Here's how the part is built. I have some questions about the finished solid (model axes, mm). Face numbers are marked on the shaded views. A direction names the side the tool comes from. Coordinates: 2 decimals unless noted, no trailing zeros. Write each loop counter-clockwise with the first axis right and the second up, starting at its lowest first coordinate (ties: lowest second). Pieces come first, ordered by that corner, then holes.
(1) Thinking about a two-plate mould opening in Z: for the marked faces 1, 2 and 3, which applies, released by +Z, released by -Z, zero draft, split by the parting line, or undercut?
(2) Please list where these lines run through material, in increasing order: probe 1 along X at (y, z) = (25, 31.2); probe 2 along Z at (x, y) = (-1, 24); probe 3 along Z at (x, y) = (-24, 35).
(3) Which directions (+Z, -Z, +X, -X, +Y, -Y) give clear straight access to the entire face, cutting with the end or side of a thin tool? Please do the marked faces 4, 5, 6 and 7.
(4) Imagine slicing it at C-C, the plane x = 14. List the corners of the cut face in (y, z) for me.
(5) Imagine slicing it at A-A, the plane x = 22. List the corners of the cut face in (y, z) for me.
(6) For pin 1 Ø24 at (x, y) = (6.5, 24.5) entering from -Z; pin 2 Ø4 at (x, z) = (-10, -23) entering from +Y; pin 3 Ø3 at (x, y) = (17, 1.5) entering from -Z (3 decimals); pin 4 Ø25 at (y, z) = (39, -11.5) entering from +X, each with a flat end and sliding along its axis, tell me the tip position at first contact or that it passes through.
(7) Imagine slicing it at D-D, the plane y = 31. List the corners of the cut face in (x, z) for me.
(8) Imagine slicing it at B-B, the plane z = 5. List the corners of the cut face in (x, y) for me.
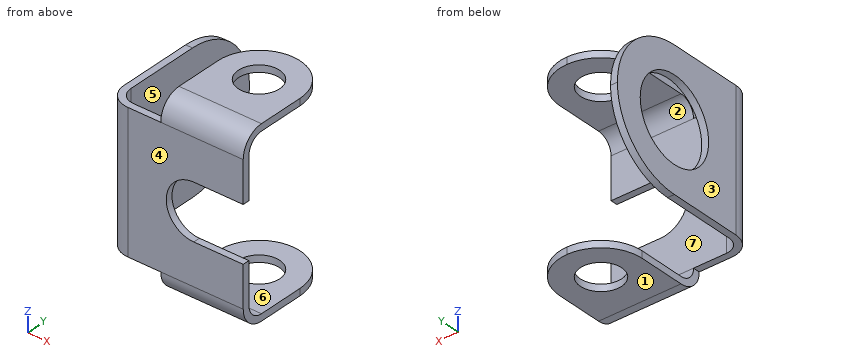
```python
from build123d import *

# Parameters (mm, degrees)
SKETCH1_W                    = 50
SKETCH1_H                    = 50
BASE_FLANGE1_DEPTH           = 2.5
EDGE_FLANGE1_STRIP_W         = 21
EDGE_FLANGE1_STRIP_H         = 2.5
EDGE_FLANGE1_STRIP_CUT_DEPTH = 50
EDGE_FLANGE1_DEPTH           = 50
BREAK_CORNER1_START          = -25
BREAK_CORNER1_DEPTH          = 2.5
SKETCH9_R                    = 15
CUT_EXTRUDE1_DEPTH           = 10
EDGE_FLANGE2_DEPTH           = 30
BREAK_CORNER2_START          = -33
BREAK_CORNER2_DEPTH          = 66
CUT_EXTRUDE2_DEPTH           = 93.633687177
CUT_EXTRUDE2_DEPTH_BACK      = 93.633687177
SKETCH13_R                   = 7.5
CUT_EXTRUDE3_DEPTH           = 71.853722556
CUT_EXTRUDE3_DEPTH_BACK      = 71.853722556


# Read off the part's stored shape, not the designer's step: Break-Corner1, Break-Corner2
# Sheet-metal steps are written as plain solids
with BuildPart() as part:
    # Sketch1 → Base-Flange1 (new body)
    with BuildSketch(Plane(origin=(0, 0, 0), x_dir=(1, 0, 0), z_dir=(0, 1, 0))):
        Rectangle(SKETCH1_W, SKETCH1_H)
    extrude(amount=BASE_FLANGE1_DEPTH)

    # Edge-Flange1 strip (across the edge) → Edge-Flange1 strip cut (cut)
    with BuildSketch(Plane(origin=(-25, 2.5, -25), x_dir=(1, 0, 0), z_dir=(0, 0, 1))):
        with Locations((-2.5, -1.25)):
            Rectangle(EDGE_FLANGE1_STRIP_W, EDGE_FLANGE1_STRIP_H)
    extrude(amount=EDGE_FLANGE1_STRIP_CUT_DEPTH, mode=Mode.SUBTRACT)

    # Edge-Flange1 section (across the edge) → Edge-Flange1 (add)
    with BuildSketch(Plane(origin=(-25, 2.5, -25), x_dir=(1, 0, 0), z_dir=(0, 0, 1))):
        with BuildLine():
            Line((0, 5.5), (0, 57.5))
            Line((0, 57.5), (2.5, 57.5))
            Line((2.5, 57.5), (2.5, 5.5))
            ThreePointArc((2.5, 5.5), (4.110912703, 1.610912703), (8, 0))
            Line((8, 0), (8, -2.5))
            ThreePointArc((8, -2.5), (2.343145751, -0.156854249), (0, 5.5))
        make_face()
    extrude(amount=EDGE_FLANGE1_DEPTH)

    # Break-Corner1 outline → Break-Corner1 (cut)
    with BuildSketch(Plane.YZ.offset(BREAK_CORNER1_START)):
        with BuildLine():
            Line((60, -25), (60, 0))
            ThreePointArc((60, 0), (52.67766953, -17.67766953), (35, -25))
            Line((35, -25), (60, -25))
        make_face()
        with BuildLine():
            ThreePointArc((35, 25), (52.67766953, 17.67766953), (60, 0))
            Line((60, 0), (60, 25))
            Line((60, 25), (35, 25))
        make_face()
    extrude(amount=BREAK_CORNER1_DEPTH, mode=Mode.SUBTRACT)

    # Sketch9 → Cut-Extrude1 (cut)
    with BuildSketch(Plane(origin=(-22.5, 0, 0), x_dir=(0, 0, -1), z_dir=(1, 0, 0))):
        with Locations(Location((0, 35, 0), (0, 0, 90))):
            Circle(SKETCH9_R)
    extrude(amount=-CUT_EXTRUDE1_DEPTH, mode=Mode.SUBTRACT)

    # Edge-Flange2 section (across the edge) → Edge-Flange2 (add)
    with BuildSketch(Plane(origin=(-5, 2.5, 30.5), x_dir=(0, 0, -1), z_dir=(1, 0, 0))):
        with BuildLine():
            Line((-2.5, 5.5), (-2.5, 37.5))
            Line((-2.5, 37.5), (0, 37.5))
            Line((0, 37.5), (0, 5.5))
            ThreePointArc((0, 5.5), (1.610912703, 1.610912703), (5.5, 0))
            Line((5.5, 0), (5.5, -2.5))
            ThreePointArc((5.5, -2.5), (-0.156854249, -0.156854249), (-2.5, 5.5))
        make_face()
    edge_flange2 = extrude(amount=EDGE_FLANGE2_DEPTH)

    # Mirror1: Edge-Flange2 across plane
    add(edge_flange2.mirror(Plane.XY))

    # Break-Corner2 outline → Break-Corner2 (cut)
    with BuildSketch(Plane.XY.offset(BREAK_CORNER2_START)):
        with BuildLine():
            ThreePointArc((-5, 25), (-0.606601718, 35.606601718), (10, 40))
            Line((10, 40), (-5, 40))
            Line((-5, 40), (-5, 25))
        make_face()
        with BuildLine():
            ThreePointArc((10, 40), (20.606601718, 35.606601718), (25, 25))
            Line((25, 25), (25, 40))
            Line((25, 40), (10, 40))
        make_face()
    extrude(amount=BREAK_CORNER2_DEPTH, mode=Mode.SUBTRACT)

    # Sketch13 → Cut-Extrude2 (cut, two sides: drawn at the far end of the back side and taken through both)
    with BuildSketch(Plane(origin=(0, 0, -33), x_dir=(-1, 0, 0), z_dir=(0, 0, -1)).offset(-CUT_EXTRUDE2_DEPTH_BACK)):
        with Locations(Location((-10, 25, 0), (0, 0, 90))):
            Circle(SKETCH13_R)
    extrude(amount=CUT_EXTRUDE2_DEPTH + CUT_EXTRUDE2_DEPTH_BACK, mode=Mode.SUBTRACT)

    # Sketch14 → Cut-Extrude3 (cut, two sides: drawn at the far end of the back side and taken through both)
    with BuildSketch(Plane(origin=(0, 2.5, 0), x_dir=(1, 0, 0), z_dir=(0, 1, 0)).offset(-CUT_EXTRUDE3_DEPTH_BACK)):
        with BuildLine():
            Line((7, 10), (37.302325581, 10))
            ThreePointArc((37.302325581, 10), (47.302325581, 0), (37.302325581, -10))
            Line((37.302325581, -10), (7, -10))
            ThreePointArc((7, -10), (-3, 0), (7, 10))
        make_face()
    extrude(amount=CUT_EXTRUDE3_DEPTH + CUT_EXTRUDE3_DEPTH_BACK, mode=Mode.SUBTRACT)


solid = part.part
```
Recorded:
1. face 1: released by -Z
1. face 2: undercut
1. face 3: zero draft
2. probe 1: x = -5 to 2.5, 17.5 to 25
2. probe 2: z = -33 to -30.5, 30.5 to 33
2. probe 3: z = -25 to -15, 15 to 25
3. face 4: +Z, -Z, +X, -X, -Y
3. face 5: +Z, -Z, +X, +Y
3. face 6: +X, -X, +Y
3. face 7: +X, +Y
4. outline: (0, -25) arc R8 ccw to (8, -33) - (18.66, -33) - (18.66, -30.5) - (8, -30.5) arc R5.5 cw to (2.5, -25) - (2.5, -10) - (0, -10) - close; (0, 10) - (2.5, 10) - (2.5, 25) arc R5.5 cw to (8, 30.5) - (18.66, 30.5) - (18.66, 33) - (8, 33) arc R8 ccw to (0, 25) - close; (31.34, -33) - (39.46, -33) - (39.46, -30.5) - (31.34, -30.5) - close; (31.34, 30.5) - (39.46, 30.5) - (39.46, 33) - (31.34, 33) - close
5. outline: (0, -25) arc R8 ccw to (8, -33) - (34, -33) - (34, -30.5) - (8, -30.5) arc R5.5 cw to (2.5, -25) - (2.5, -10) - (0, -10) - close; (0, 10) - (2.5, 10) - (2.5, 25) arc R5.5 cw to (8, 30.5) - (34, 30.5) - (34, 33) - (8, 33) arc R8 ccw to (0, 25) - close
6. pin 1: stops at z = -33
6. pin 2: stops at y = 2.5
6. pin 3: stops at z = -31.245
6. pin 4: stops at x = -22.5
7. outline: (-25, -25) - (-22.5, -25) - (-22.5, -14.46) - (-25, -14.46) - close; (-25, 14.46) - (-22.5, 14.46) - (-22.5, 25) - (-25, 25) - close; (-3.75, -33) - (5.5, -33) - (5.5, -30.5) - (-3.75, -30.5) - close; (-3.75, 30.5) - (5.5, 30.5) - (5.5, 33) - (-3.75, 33) - close; (14.5, -33) - (23.75, -33) - (23.75, -30.5) - (14.5, -30.5) - close; (14.5, 30.5) - (23.75, 30.5) - (23.75, 33) - (14.5, 33) - close
8. outline: (-25, 8) arc R8 ccw to (-17, 0) - (-1.66, 0) - (-1.66, 2.5) - (-17, 2.5) arc R5.5 cw to (-22.5, 8) - (-22.5, 20.86) - (-25, 20.86) - close; (-25, 49.14) - (-22.5, 49.14) - (-22.5, 59.49) - (-25, 59.49) - close
